Read the model definition and answer for the solid it produces. Units are mm, in the model's axes. A direction names the side the tool comes from. Coordinates: 2 decimals unless noted, no trailing zeros. Order: outer loops, then holes, each group sorted by start corner. A loop starts at its lowest first (then second) coordinate and runs counter-clockwise, first axis right, second up. Notation, with made-up numbers: M 47.25,40.5 L 51.25,40.5 A32 cw 51.25,70.5 Z; hole C 40,84.5 d4. An arc over 180 degrees is marked long. Use a Markdown table: item, result. Add a question column.
1) Find section A-A on y = 3. Write down the section's boundary in (x, z).
2) For faces 1 (the face through (0.8, -3.18, -1.05)), 2 (the face through (0, 1.5, 1)), 3 (the face through (-2.083, 3.9, 2.5)), 4 (the face through (2.5, 3.9, -2.083)), determine the directions among +Z, -Z, +X, -X, +Y, -Y from which every point of the face is accessible in a straight line to the end or side of a thin tool.
3) Find the intervals of material crossed by probe 1 along X at (y, z) = (5, 2.75); probe 2 along X at (y, z) = (-2, 0), in increasing order. Write a range as [from, to].
4) The mould has two halves that part along Z. Classify faces 5 (the face through (0, 1, 2.997)), 6 (the face through (0, 0, 0)), 7 (the face through (2.083, 3.9, -2.5)), 8 (the face through (-2.5, 3.9, -2.083)): released by +Z, released by -Z, zero draft, split by the parting line, or undercut.
5) Find section D-D on y = -4.75. Write down the section's boundary in (x, z).
from build123d import *

# Parameters (mm, degrees)
SKETCH1_W           = 5.9944
SKETCH1_H           = 5.9944
BOSS_EXTRUDE1_DEPTH = 1.5
SKETCH2_W           = 1.6764
SKETCH2_H           = 1.6764
BOSS_EXTRUDE2_DEPTH = 0.5
SKETCH3_W           = 0.9144
SKETCH3_H           = 0.9144
BOSS_EXTRUDE3_DEPTH = 3.937
SKETCH4_R           = 2.7472
SKETCH4_R_2         = 1.3208
BOSS_EXTRUDE4_DEPTH = 6.5852
CHAMFER1_SIZE       = 0.125
SKETCH7_R           = 0.4826
BOSS_EXTRUDE5_DEPTH = 4.437
CHAMFER2_SIZE       = 0.25


with BuildPart() as part:
    # Sketch1 → Boss-Extrude1 (new body)
    with BuildSketch(Plane(origin=(0, 0, 0), x_dir=(1, 0, 0), z_dir=(0, 1, 0))):
        Rectangle(SKETCH1_W, SKETCH1_H)
    extrude(amount=BOSS_EXTRUDE1_DEPTH)

    # Sketch2 → Boss-Extrude2 (add)
    with BuildSketch(Plane(origin=(0, 1.5, 0), x_dir=(1, 0, 0), z_dir=(0, 1, 0))):
        with Locations((-2.159, 2.159)):
            Rectangle(SKETCH2_W, SKETCH2_H)
        with Locations((2.159, 2.159)):
            Rectangle(SKETCH2_W, SKETCH2_H)
        with Locations((2.159, -2.159)):
            Rectangle(SKETCH2_W, SKETCH2_H)
        with Locations((-2.159, -2.159)):
            Rectangle(SKETCH2_W, SKETCH2_H)
    extrude(amount=BOSS_EXTRUDE2_DEPTH)

    # Sketch3 → Boss-Extrude3 (add)
    with BuildSketch(Plane(origin=(0, 2, 0), x_dir=(1, 0, 0), z_dir=(0, 1, 0))):
        with Locations((-2.54, -2.54)):
            Rectangle(SKETCH3_W, SKETCH3_H)
        with Locations((2.54, -2.54)):
            Rectangle(SKETCH3_W, SKETCH3_H)
        with Locations((2.54, 2.54)):
            Rectangle(SKETCH3_W, SKETCH3_H)
        with Locations((-2.54, 2.54)):
            Rectangle(SKETCH3_W, SKETCH3_H)
    extrude(amount=BOSS_EXTRUDE3_DEPTH)

    # Sketch4 → Boss-Extrude4 (add)
    with BuildSketch(Plane.XZ):
        with Locations(Location((0, 0, 0), (0, 0, 90))):
            Circle(SKETCH4_R)
        with Locations(Location((0, 0, 0), (0, 0, 90))):
            Circle(SKETCH4_R_2, mode=Mode.SUBTRACT)
    extrude(amount=BOSS_EXTRUDE4_DEPTH)

    # Chamfer1
    chamfer1_edges = [part.edges().sort_by_distance(p)[0] for p in [
        (0, -6.5852, -1.3208),
        (0, -6.5852, -2.7472),
    ]]
    chamfer(chamfer1_edges, length=CHAMFER1_SIZE)

    # Sketch5 → Cut-Revolve1 (revolve, cut)
    with BuildSketch(Plane.XY, mode=Mode.PRIVATE) as cut_revolve1_sk:
        with BuildLine():
            Line((-2.7472, 0), (-2.7472, -1.524))
            Line((-2.7472, -1.524), (-2.3828, -1.8884))
            Line((-2.3828, -1.8884), (-2.3828, -2.0384))
            Line((-2.3828, -2.0384), (-2.122992379, -2.4884))
            Line((-2.122992379, -2.4884), (-1.822992379, -2.4884))
            Line((-1.822992379, -2.4884), (-1.822992379, -5.330737835))
            ThreePointArc((-1.822992379, -5.330737835), (-2.0828, -5.957968917), (-1.822992379, -6.5852))
            Line((-1.822992379, -6.5852), (-3.193096247, -6.5852))
            Line((-3.193096247, -6.5852), (-3.193096247, 0))
            Line((-3.193096247, 0), (-2.7472, 0))
        make_face()
    revolve(cut_revolve1_sk.sketch.rotate(Axis((0, -6.4602, 0), (0, 1, 0)), 270), axis=Axis((0, -6.4602, 0), (0, 1, 0)), mode=Mode.SUBTRACT)

    # Sketch7 → Boss-Extrude5 (add)
    with BuildSketch(Plane(origin=(0, 1.5, 0), x_dir=(1, 0, 0), z_dir=(0, 1, 0))):
        with Locations(Location((0, 0, 0), (0, 0, 90))):
            Circle(SKETCH7_R)
    extrude(amount=BOSS_EXTRUDE5_DEPTH)

    # Chamfer2
    chamfer2_edges = [part.edges().sort_by_distance(p)[0] for p in [
        (0, 5.937, 0.4826),
    ]]
    chamfer(chamfer2_edges, length=CHAMFER2_SIZE)


solid = part.part
Check result:
| question | item | result |
|---|---|---|
| 1 | outline | M -3,-3 L -2.08,-3 L -2.08,-2.08 L -3,-2.08 Z; M -3,2.08 L -2.08,2.08 L -2.08,3 L -3,3 Z; C 0,0 d0.97; M 2.08,-3 L 3,-3 L 3,-2.08 L 2.08,-2.08 Z; M 2.08,2.08 L 3,2.08 L 3,3 L 2.08,3 Z |
| 2 | face 1 | -Y |
| 2 | face 2 | +Y |
| 2 | face 3 | +Z, -Z, +Y |
| 2 | face 4 | +X, -X, +Y |
| 3 | probe 1 | x = [-3, -2.08], [2.08, 3] |
| 3 | probe 2 | x = [-2.38, -1.32], [1.32, 2.38] |
| 4 | face 5 | released by +Z |
| 4 | face 6 | undercut |
| 4 | face 7 | zero draft |
| 4 | face 8 | undercut |
| 5 | outline | C 0,0 d3.65; hole C 0,0 d2.64 |
